Check sheet for the drawn part. Datum: minimum x, y, z corner. Units: mm. A direction names the side the tool comes from. Give positions to 0.01 mm unless a question says otherwise; leave off trailing zeros. Loops run counter-clockwise (first coordinate to the right, second up) from the corner with the lowest first, then second, coordinate; pieces in that order, holes last. Notation, with made-up numbers: M 63.5,-3 L 93.5,-3 A28 ccw 93.5,33 Z; hole C 72,-20 d4. An arc over 180 degrees is marked long. Write each question's results on one line, items separated by ' | '. Start each with the question number.
1. Material ranges on line 1 along Y through (x, z) = (15.5, 9.5) (1 decimal); line 2 along Y through (x, z) = (28, 24); line 3 along X through (y, z) = (20.5, 48.5) (1 decimal), recorded low to high.
2. Go/stop test with flat-tipped pins: pin 1 (6 mm diameter, centred on x = 4.5, z = 23, fed in from -Y) (1 decimal); pin 2 (3.5 mm diameter, centred on y = 25.5, z = 18, fed in from -X); pin 3 (2.5 mm diameter, centred on x = 3, z = 22, fed in from +Y). Record where each tip stops, or that it passes through.
3. Draft check along Z on the marked faces 4, 5 and 6. Enter one of: pulls with the +Z half, pulls with the -Z half, needs draft (parallel to the pull), parting line crosses it, or undercut.
4. Sectioned sample at B-B on y = 26.5. Record the cut outline in (x, z) (1 decimal).
5. Sectioned sample at C-C on x = 4. Record the cut outline in (y, z).
6. Tool access check on the marked faces 1, 2 and 3. Record the directions out of +Z, -Z, +X, -X, +Y, -Y that give a thin tool (end or side, any length) a straight path to the whole face; none if there is none.
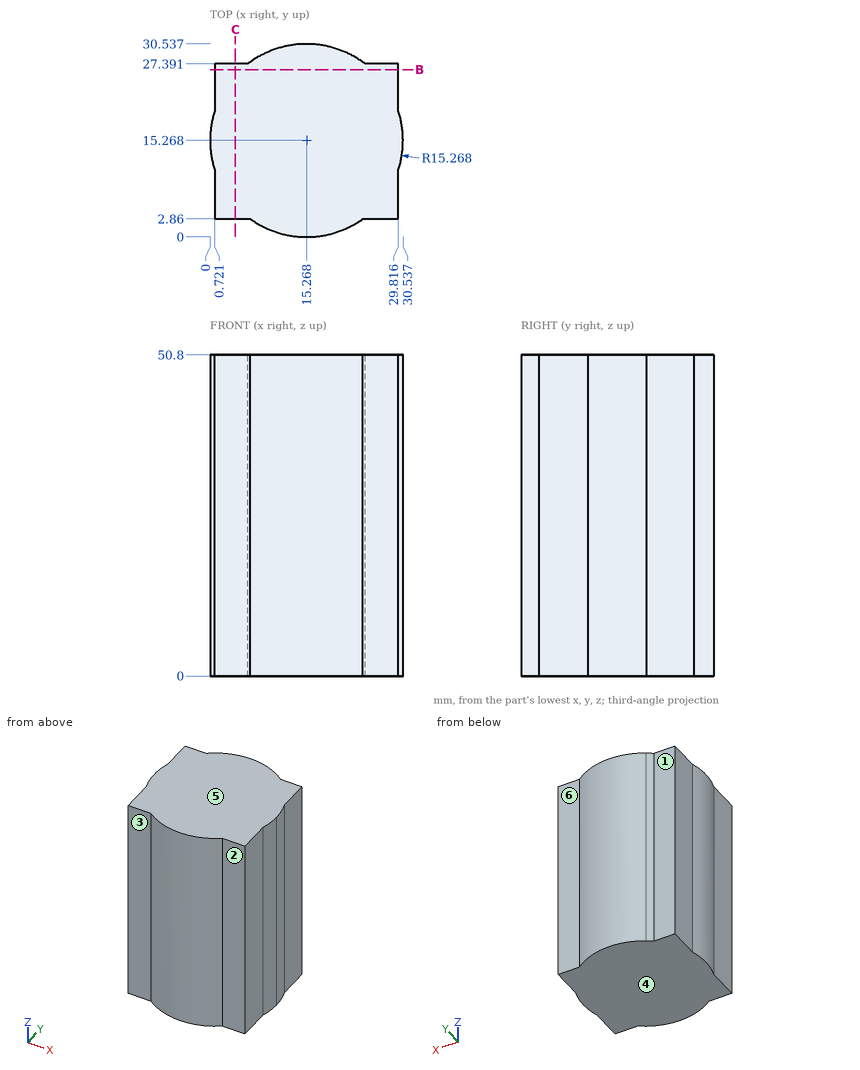
Output values:
1) line 1: 0 to 30.5 | line 2: 2.86 to 27.39 | line 3: 0.7 to 29.8
2) pin 1: y = 2.1 | pin 2: x = 0.72 | pin 3: y = 27.39
3) face 4: pulls with the -Z half | face 5: pulls with the +Z half | face 6: needs draft
4) outline: M 0.7,0 L 29.8,0 L 29.8,50.8 L 0.7,50.8 Z
5) outline: M 2.86,0 L 27.39,0 L 27.39,50.8 L 2.86,50.8 Z
6) face 1: +Z, -Z, -X, +Y | face 2: +Z, -Z, +X, -Y | face 3: +Z, -Z, -X, -Y
